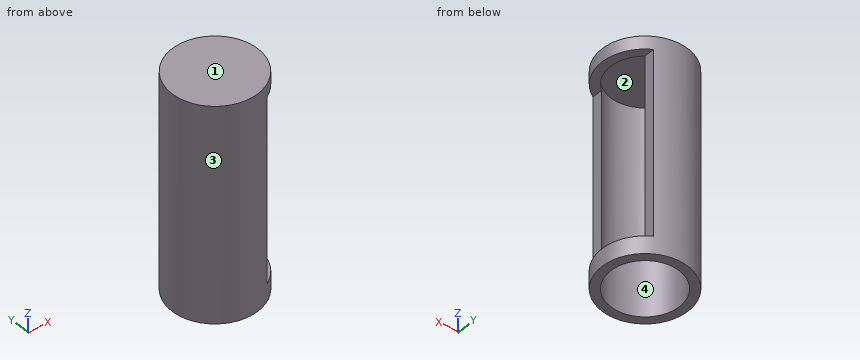
from build123d import *

# Parameters (mm, degrees)
F0_R     = 12.7
F1_DEPTH = 63.82626
F3_T     = -2.54
F4_W     = 43.020739
F4_H     = 54.811081
F5_DEPTH = 45.41777
F2_W     = 40.954981
F2_H     = 44.655449
F6_DEPTH = 29.8618


with BuildPart() as f1:
    # F0 (on Top) → F1 (new body)
    with BuildSketch(Plane.XY):
        with Locations((-51.784314, 43.91994)):
            Circle(F0_R)
    extrude(amount=F1_DEPTH)

    # F3
    f3_openings = [f1.faces().sort_by_distance(p)[0] for p in [
        (-51.784314, 43.91994, 0),
    ]]
    offset(amount=F3_T, openings=f3_openings)

    # F4 (on Right) → F5 (cut)
    with BuildSketch(Plane.YZ):
        with Locations((47.886142, 32.577515)):
            Rectangle(F4_W, F4_H)
    extrude(amount=-F5_DEPTH, mode=Mode.SUBTRACT)

    # F2 (on Front) → F6 (cut)
    with BuildSketch(Plane.XZ):
        with Locations((-53.447423, 32.679513)):
            Rectangle(F2_W, F2_H)
    extrude(amount=-F6_DEPTH, mode=Mode.SUBTRACT)


solid = f1.part
The listing builds one solid part. Answer for the finished solid, in the listing's coordinates (mm). Face numbers are marked on the shaded views. Round coordinates to 2 decimals unless told otherwise and drop trailing zeros. Order: outer loops, then holes, each group sorted by start corner. A loop starts at its lowest first (then second) coordinate and runs counter-clockwise, first axis right, second up. Notation, with made-up numbers: (57, 66.5) -> (99, 66.5) arc R16 cw to (99, 72.5) -> close; hole circle Ø3 at (66.5, 39.5). An arc over 180 degrees is marked (long way). Write each question's results on one line, items separated by ' | '. Start each with the question number.
Q1. Straight lines are drawn through the part: probe 1 along Z at (x, y) = (-41.75, 38.5); probe 2 along Y at (x, z) = (-51.5, 13.5); probe 3 along Z at (x, y) = (-59.75, 43). For each, find the intervals that lie inside material, in ascending order. Write a range as from..to.
Q2. Find section C-C (y = 34.5). Determine the outline of the cut face in (x, z).
Q3. Find section B-B (y = 39). Determine the outline of the cut face in (x, z) (3 decimals), then the cut area to 3 significant figures.
Q4. The mould has two halves that part along X. Classify the marked faces 1, 2, 3 and 4: pulls with the +X half, pulls with the -X half, needs draft (parallel to the pull), parting line crosses it, or undercut.
Q5. Each of these flat-tipped pins is pushed along its axis until it touches: pin 1 (4 mm diameter, centred on y = 48, z = 10.5, fed in from +X); pin 2 (0.9 mm diameter, centred on y = 35, z = 29.5, fed in from +X); pin 3 (4 mm diameter, centred on x = -49, z = 53, fed in from -Y). Where does it stop, or does it pass through?
Q6. Find section A-A (x = -40.75). Determine the outline of the cut face in (y, z), then the cut area to 3 significant figures.
Q7. Find section D-D (x = -47.5). Determine the outline of the cut face in (y, z), then the cut area to 3 significant figures.
Worked answers:
1) probe 1: z = 0..5.17, 59.98..63.83 | probe 2: y = 31.22..33.76, 54.08..56.62 | probe 3: z = 61.29..63.83
2) outline: (-60.3, 0) -> (-55.59, 0) -> (-55.59, 61.29) -> (-47.98, 61.29) -> (-47.98, 0) -> (-43.27, 0) -> (-43.27, 5.17) -> (-45.42, 5.17) -> (-45.42, 59.98) -> (-43.27, 59.98) -> (-43.27, 63.83) -> (-60.3, 63.83) -> close
3) outline: (-63.493, 0) -> (-60.674, 0) -> (-60.674, 61.286) -> (-42.895, 61.286) -> (-42.895, 59.983) -> (-40.076, 59.983) -> (-40.076, 63.826) -> (-63.493, 63.826) -> close; (-42.895, 0) -> (-40.076, 0) -> (-40.076, 5.172) -> (-42.895, 5.172) -> close | area: 250 mm2
4) face 1: needs draft | face 2: undercut | face 3: parting line crosses it | face 4: undercut
5) pin 1: stops at x = -59.92 | pin 2: stops at x = -45.42 | pin 3: stops at y = 31.24
6) outline: (37.63, 0) -> (50.21, 0) -> (50.21, 5.17) -> (37.63, 5.17) -> close; (37.63, 59.98) -> (50.21, 59.98) -> (50.21, 63.83) -> (37.63, 63.83) -> close | area: 113 mm2
7) outline: (31.96, 0) -> (34.71, 0) -> (34.71, 61.29) -> (53.13, 61.29) -> (53.13, 0) -> (55.88, 0) -> (55.88, 63.83) -> (31.96, 63.83) -> close | area: 397 mm2
